```python
from build123d import *

# Parameters (mm, degrees)
ESQUISSE1_W          = 6
ESQUISSE1_H          = 6
BASE_EXTRUSION_DEPTH = 60
CONG_1_R             = 3


with BuildPart() as part:
    # Esquisse1 → Base-Extrusion (new body)
    with BuildSketch(Plane.XY):
        with Locations((3, 3)):
            Rectangle(ESQUISSE1_W, ESQUISSE1_H)
    extrude(amount=BASE_EXTRUSION_DEPTH)

    # Congé1
    cong_1_edges = [part.edges().sort_by_distance(p)[0] for p in [
        (6, 3, 0),
        (6, 3, 60),
        (0, 3, 0),
        (0, 3, 60),
    ]]
    fillet(cong_1_edges, radius=CONG_1_R - 0.0001)  # a hair under: the kernel refuses the full size


solid = part.part
```
Here's how the part is built. I have some questions about the finished solid (model axes, mm). Coordinates: 2 decimals unless noted, no trailing zeros. Order: outer loops, then holes, each group sorted by start corner. A loop starts at its lowest first (then second) coordinate and runs counter-clockwise, first axis right, second up. Notation, with made-up numbers: (17, 5.25) - (39, 5.25) arc R17 ccw to (39, 19.25) - close; hole circle Ø1 at (51.5, 10). An arc over 180 degrees is marked (long way). One line per question, with ' | ' between items. Start each with the question number.
1. If we section it at B-B (x = 1.35): Write out the boundary of the cut face in (y, z).
2. If we section it at C-C (x = 5.3): Write out the boundary of the cut face in (y, z).
3. Please list where these lines run through material, in increasing order: line 1 along Z through (x, y) = (2.9, 3.4); line 2 along Z through (x, y) = (4.95, 3.15); line 3 along X through (y, z) = (5, 2). Write a range as [from, to].
Model answer:
1) outline: (0, 0.49) - (6, 0.49) - (6, 59.51) - (0, 59.51) - close
2) outline: (0, 1.07) - (6, 1.07) - (6, 58.93) - (0, 58.93) - close
3) line 1: z = [0, 60] | line 2: z = [0.72, 59.28] | line 3: x = [0.17, 5.83]
